Geometry: final body of the model. Coordinates: model frame, mm. A direction names the side the tool comes from. Give positions to 0.01 mm unless a question says otherwise; leave off trailing zeros. Write each loop counter-clockwise with the first axis right and the second up, starting at its lowest first coordinate (ties: lowest second). Pieces come first, ordered by that corner, then holes. Notation, with made-up numbers: M 32.5,34.25 L 53.5,34.25 A10 ccw 53.5,49.25 Z; hole C -25.75,-3 d5. An arc over 180 degrees is marked long. Use a Markdown table: item, result. Add a question column.
1) Pin query (flat end, axial travel): pin 1 (20 mm diameter, centred on x = 5, y = -14.5, fed in from +Z); pin 2 (3 mm diameter, centred on y = -0.5, z = 8, fed in from +X); pin 3 (5 mm diameter, centred on y = -18.5, z = 9.1, fed in from -X); pin 4 (12 mm diameter, centred on y = 16.5, z = 10.5, fed in from -X). Return the tip coordinate at first contact, or that it passes through.
2) Line query: line 1 (Y direction, x = 15, z = 12.25); line 2 (X direction, y = 24.5, z = 6.25); line 3 (Y direction, x = 29.5, z = 14.75). Output: solid intervals per line, ascending.
3) Section D-D on z = 9. State how many separate pieces and enclosed holes the cut face has, then the cut area to 3 significant figures.
4) Section B-B on z = 3.5. Return the cut outline in (x, y).
5) Section C-C on y = 24. Return the cut outline in (x, z), then the cut area to 3 significant figures.
6) Draft query along X for faces 1 (the flat face through (-34.5, 0, 4)), 2 (the flat face through (34, -1, 8)), 3 (the cylindrical face through (33.26, 0.055, 10.345)), 4 (the flat face through (32.5, 0, 12)). Return one class per face: +X half, -X half, draft (parallel to the pull), parting line (faces both ways), or undercut.
7) Set-up query: faces 5 (the flat face through (0, -9, 9)), 6 (the cylindrical face through (34.25, -21.43, 9.75)), 7 (the cylindrical face through (-34.25, -21.43, 9.75)), 8 (the flat face through (0, 28, 8)). Return all of +Z, -Z, +X, -X, +Y, -Y with unobstructed straight access to the full face (end or side cutting, diameter ignored); none if empty.
8) Section A-A on y = 0. Return the cut outline in (x, z).
```python
from build123d import *

# Parameters (mm, degrees)
SKETCH2_W           = 69
SKETCH2_H           = 60
SKETCH2_W_2         = 65
SKETCH2_H_2         = 56
BOSS_EXTRUDE1_DEPTH = 19
SKETCH3_W           = 69
SKETCH3_H           = 60
BOSS_EXTRUDE2_DEPTH = 1
BOSS_EXTRUDE4_DEPTH = 67.5
CUT_EXTRUDE1_DEPTH  = 135
SKETCH7_W           = 84.404027411
SKETCH7_H           = 26.874448114
CUT_EXTRUDE2_DEPTH  = 135
SKETCH9_W           = 65
SKETCH9_H           = 1
BOSS_EXTRUDE5_DEPTH = 17
FILLET1_R           = 1
SKETCH10_R          = 3
CUT_EXTRUDE6_DEPTH  = 0.5
CUT_EXTRUDE7_REACH  = 79.602
SKETCH11_R          = 1.25


with BuildPart() as part:
    # Sketch2 → Boss-Extrude1 (new body)
    with BuildSketch(Plane.XY):
        Rectangle(SKETCH2_W, SKETCH2_H)
        Rectangle(SKETCH2_W_2, SKETCH2_H_2, mode=Mode.SUBTRACT)
    extrude(amount=BOSS_EXTRUDE1_DEPTH)

    # Sketch3 → Boss-Extrude2 (add, symmetric)
    with BuildSketch(Plane(origin=(0, 0, 0), x_dir=(-1, 0, 0), z_dir=(0, 0, -1))):
        Rectangle(SKETCH3_W, SKETCH3_H)
    extrude(amount=BOSS_EXTRUDE2_DEPTH, both=True)

    # Sketch4 → Boss-Extrude4 (add, symmetric)
    with BuildSketch(Plane.ZY.offset(34.5)):
        with BuildLine():
            Line((19, -27.062112177), (17.917720438, -26.385779399))
            add(Edge.make_bspline(
                [(17.917720438, -26.385779399), (17.068052287, -28.229247979), (14.940376438, -27.841186756), (13.351451557, -28.086320914)],
                knots=[0, 0, 0, 0, 1, 1, 1, 1], degree=3))
            Line((13.351451557, -28.086320914), (14.231772034, -30))
            add(Edge.make_bspline(
                [(14.231772034, -30), (17.788479479, -29.104156819), (19, -27.062112177)],
                knots=[0, 0, 0, 0.719469437, 0.719469437, 0.719469437], degree=2))
        make_face()
        with BuildLine():
            Line((14.231772034, 30), (13.351451557, 28.086320914))
            add(Edge.make_bspline(
                [(17.917720438, 26.385779399), (17.068052287, 28.229247979), (14.940376438, 27.841186756), (13.351451557, 28.086320914)],
                knots=[0, 0, 0, 0, 1, 1, 1, 1], degree=3))
            Line((17.917720438, 26.385779399), (19, 27.062112177))
            add(Edge.make_bspline(
                [(14.231772034, 30), (17.788479479, 29.104156819), (19, 27.062112177)],
                knots=[0, 0, 0, 0.719469437, 0.719469437, 0.719469437], degree=2))
        make_face()
    extrude(amount=BOSS_EXTRUDE4_DEPTH, both=True)

    # Sketch6 → Cut-Extrude1 (cut)
    with BuildSketch(Plane.ZY.offset(34.5)):
        Polygon((19, -30), (19, -27.062112177), (18.840520093, -27.311263152), (18.318412732, -27.941049653), (17.662350265, -28.50734155), (16.534506271, -29.184167719), (14.231772034, -30), align=None)
        Polygon((19, 30), (14.231772034, 30), (16.534506271, 29.184167719), (17.662350265, 28.50734155), (18.318412732, 27.941049653), (18.840520093, 27.311263152), (19, 27.062112177), align=None)
    extrude(amount=-CUT_EXTRUDE1_DEPTH, mode=Mode.SUBTRACT)

    # Sketch7 → Cut-Extrude2 (cut)
    with BuildSketch(Plane.XZ.offset(30)):
        with Locations((-76.702013706, 12.437224057)):
            Rectangle(SKETCH7_W, SKETCH7_H)
    extrude(amount=-CUT_EXTRUDE2_DEPTH, mode=Mode.SUBTRACT)

    # Sketch9 → Boss-Extrude5 (add)
    with BuildSketch(Plane.XY.offset(1)):
        with Locations((0, 9.5)):
            Rectangle(SKETCH9_W, SKETCH9_H)
        with Locations((0, -9.5)):
            Rectangle(SKETCH9_W, SKETCH9_H)
    extrude(amount=BOSS_EXTRUDE5_DEPTH)

    # Fillet1
    fillet1_edges = [part.edges().sort_by_distance(p)[0] for p in [
        (-34.5, 30, 6.615886017),
        (-34.5, -30, 6.615886017),
        (34.5, 30, 6.615886017),
        (34.5, -30, 6.615886017),
    ]]
    fillet(fillet1_edges, radius=FILLET1_R)

    # Sketch10 → Cut-Extrude6 (cut)
    with BuildSketch(Plane(origin=(34.5, 0, 0), x_dir=(0, 0, -1), z_dir=(1, 0, 0))):
        with Locations((-9.09656972, -18.5)):
            Circle(SKETCH10_R)
        with Locations((-9.09656972, 0)):
            Circle(SKETCH10_R)
        with Locations((-9.09656972, 18.5)):
            Circle(SKETCH10_R)
    cut_extrude6 = extrude(amount=-CUT_EXTRUDE6_DEPTH, mode=Mode.SUBTRACT)

    # Cut-Extrude7: up to this face of the body (flat: up to its plane)
    cut_extrude7_end = Plane(part.part.faces().sort_by_distance((-34.5, 0, 8.972249648))[0])
    # Sketch11 → Cut-Extrude7 (cut, up to the picked face)
    with BuildSketch(Plane(origin=(34.5, 0, 0), x_dir=(0, 0, -1), z_dir=(1, 0, 0)), mode=Mode.PRIVATE) as cut_extrude7_sk1:
        with Locations((-9.09656972, -18.5)):
            Circle(SKETCH11_R)
    cut_extrude7_tool1 = split(extrude(cut_extrude7_sk1.sketch, amount=-CUT_EXTRUDE7_REACH, mode=Mode.PRIVATE), bisect_by=cut_extrude7_end, keep=Keep.BOTH, mode=Mode.PRIVATE)
    # Sketch11 → Cut-Extrude7 (cut, up to the picked face)
    with BuildSketch(Plane(origin=(34.5, 0, 0), x_dir=(0, 0, -1), z_dir=(1, 0, 0)), mode=Mode.PRIVATE) as cut_extrude7_sk2:
        with Locations((-9.09656972, 0)):
            Circle(SKETCH11_R)
    cut_extrude7_tool2 = split(extrude(cut_extrude7_sk2.sketch, amount=-CUT_EXTRUDE7_REACH, mode=Mode.PRIVATE), bisect_by=cut_extrude7_end, keep=Keep.BOTH, mode=Mode.PRIVATE)
    # Sketch11 → Cut-Extrude7 (cut, up to the picked face)
    with BuildSketch(Plane(origin=(34.5, 0, 0), x_dir=(0, 0, -1), z_dir=(1, 0, 0)), mode=Mode.PRIVATE) as cut_extrude7_sk3:
        with Locations((-9.09656972, 18.5)):
            Circle(SKETCH11_R)
    cut_extrude7_tool3 = split(extrude(cut_extrude7_sk3.sketch, amount=-CUT_EXTRUDE7_REACH, mode=Mode.PRIVATE), bisect_by=cut_extrude7_end, keep=Keep.BOTH, mode=Mode.PRIVATE)
    add(cut_extrude7_tool1.solids().sort_by(Axis((34.5, -18.5, 9.09657), (-1, 0, 0)))[0], mode=Mode.SUBTRACT)
    add(cut_extrude7_tool2.solids().sort_by(Axis((34.5, 0, 9.09657), (-1, 0, 0)))[0], mode=Mode.SUBTRACT)
    add(cut_extrude7_tool3.solids().sort_by(Axis((34.5, 18.5, 9.09657), (-1, 0, 0)))[0], mode=Mode.SUBTRACT)

    # Mirror1: Cut-Extrude6 across plane
    add(cut_extrude6.mirror(Plane(origin=(0, 0, 0), x_dir=(0, 0, 1), z_dir=(1, 0, 0))), mode=Mode.SUBTRACT)


solid = part.part
```
Found:
| question | item | result |
|---|---|---|
| 1 | pin 1 | z = 18 |
| 1 | pin 2 | x = 34 |
| 1 | pin 3 | x = -34 |
| 1 | pin 4 | x = -34.5 |
| 2 | line 1 | -30 to -28, -10 to -9, 9 to 10, 28 to 30 |
| 2 | line 2 | -34.5 to -32.5, 32.5 to 34.5 |
| 2 | line 3 | -29.82 to -27.97, -10 to -9, 9 to 10, 27.97 to 29.82 |
| 3 | separate pieces | 4 |
| 3 | enclosed holes | 0 |
| 3 | area | 589 mm² |
| 4 | outline | M -34.5,-29 A1 ccw -33.5,-30 L 33.5,-30 A1 ccw 34.5,-29 L 34.5,29 A1 ccw 33.5,30 L -33.5,30 A1 ccw -34.5,29 Z; hole M -32.5,-28 L 32.5,-28 L 32.5,-10 L -32.5,-10 Z; hole M -32.5,-9 L 32.5,-9 L 32.5,9 L -32.5,9 Z; hole M -32.5,10 L 32.5,10 L 32.5,28 L -32.5,28 Z |
| 5 | outline | M -34.5,-1 L 34.5,-1 L 34.5,19 L 32.5,19 L 32.5,1 L -32.5,1 L -32.5,19 L -34.5,19 Z |
| 5 | area | 210 mm² |
| 6 | face 1 | -X half |
| 6 | face 2 | +X half |
| 6 | face 3 | draft |
| 6 | face 4 | undercut |
| 7 | face 5 | +Z |
| 7 | face 6 | +X |
| 7 | face 7 | -X |
| 7 | face 8 | none |
| 8 | outline | M -34.5,-1 L 34.5,-1 L 34.5,6.1 L 34,6.1 L 34,7.85 L 32.5,7.85 L 32.5,1 L -32.5,1 L -32.5,7.85 L -34,7.85 L -34,6.1 L -34.5,6.1 Z; M -34.5,12.1 L -34,12.1 L -34,10.35 L -32.5,10.35 L -32.5,19 L -34.5,19 Z; M 32.5,10.35 L 34,10.35 L 34,12.1 L 34.5,12.1 L 34.5,19 L 32.5,19 Z |
